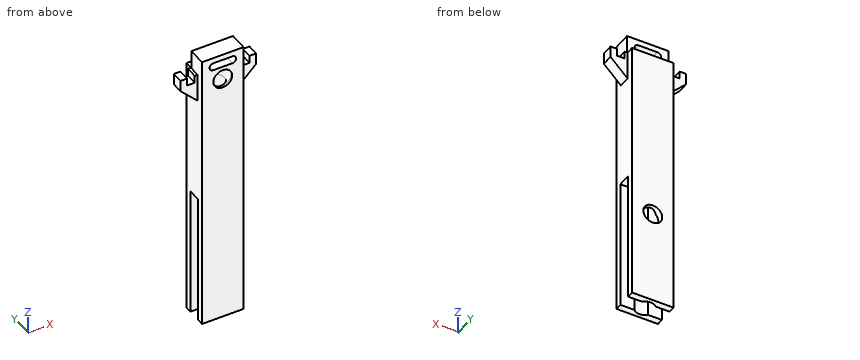
from build123d import *

# Parameters (mm, degrees)
SKETCH1_W           = 11
SKETCH1_H           = 76
BOSS_EXTRUDE1_DEPTH = 7
SKETCH4_R           = 2.5
SKETCH5_W           = 3
SKETCH5_H           = 3
BOSS_EXTRUDE2_DEPTH = 4.5
SKETCH6_W           = 2
SKETCH6_H           = 3
CUT_EXTRUDE2_DEPTH  = 2
BOSS_EXTRUDE3_DEPTH = 3
SKETCH10_W          = 11
SKETCH10_H          = 3.5
CUT_EXTRUDE5_DEPTH  = 35
CUT_EXTRUDE6_REACH  = 41.912
SKETCH11_R          = 2.5
SKETCH12_W          = 11
SKETCH12_H          = 2.25
CUT_EXTRUDE9_DEPTH  = 5
CUT_EXTRUDE10_REACH = 41.58


with BuildPart() as part:
    # Sketch1 → Boss-Extrude1 (new body)
    with BuildSketch(Plane(origin=(0, 0, 0), x_dir=(1, 0, 0), z_dir=(0, 1, 0))):
        Rectangle(SKETCH1_W, SKETCH1_H)
    extrude(amount=BOSS_EXTRUDE1_DEPTH)

    # Cut-Sweep2: sweep along a path in Sketch3
    with BuildLine(Plane.ZY) as cut_sweep2_path:
        Line((-38, 3.5), (28, 3.5))
        ThreePointArc((28, 3.5), (30.121320344, 2.621320344), (31, 0.5))
        Line((31, 0.5), (31, 0))
    # Sketch4 → Cut-Sweep2 (sweep, cut)
    with BuildSketch(Plane(origin=(0, 0, -38), x_dir=(-1, 0, 0), z_dir=(0, 0, -1))):
        with Locations((0, 3.5)):
            Circle(SKETCH4_R)
    sweep(path=cut_sweep2_path.line, mode=Mode.SUBTRACT)

    # Sketch5 → Boss-Extrude2 (add)
    with BuildSketch(Plane.ZY.offset(5.5)):
        with Locations((31.5, 3.5)):
            Rectangle(SKETCH5_W, SKETCH5_H)
    boss_extrude2 = extrude(amount=BOSS_EXTRUDE2_DEPTH)

    # Mirror1: Boss-Extrude2 across plane
    add(boss_extrude2.mirror(Plane.ZY))

    # Sketch6 → Cut-Extrude2 (cut)
    with BuildSketch(Plane.XY.offset(33)):
        with Locations((-7.25, 3.5)):
            Rectangle(SKETCH6_W, SKETCH6_H)
    cut_extrude2 = extrude(amount=-CUT_EXTRUDE2_DEPTH, mode=Mode.SUBTRACT)

    # Mirror2: Cut-Extrude2 across plane
    add(cut_extrude2.mirror(Plane.ZY), mode=Mode.SUBTRACT)

    # Sketch7 → Boss-Extrude3 (add)
    with BuildSketch(Plane(origin=(0, 5, 0), x_dir=(1, 0, 0), z_dir=(0, 1, 0))):
        Polygon((-10, -30), (-5.5, -25.5), (-5.5, -30), align=None)
    boss_extrude3 = extrude(amount=-BOSS_EXTRUDE3_DEPTH)

    # Mirror3: Boss-Extrude3 across plane
    add(boss_extrude3.mirror(Plane.ZY))

    # Sketch10 → Cut-Extrude5 (cut)
    with BuildSketch(Plane(origin=(0, 0, -38), x_dir=(-1, 0, 0), z_dir=(0, 0, -1))):
        with Locations((0, 3.5)):
            Rectangle(SKETCH10_W, SKETCH10_H)
    extrude(amount=-CUT_EXTRUDE5_DEPTH, mode=Mode.SUBTRACT)

    # Sketch11 → Cut-Extrude6 (cut, up to next)
    with BuildSketch(Plane(origin=(0, 7, 0), x_dir=(1, 0, 0), z_dir=(0, 1, 0)), mode=Mode.PRIVATE) as cut_extrude6_sk1:
        with Locations(Location((0, 13, 0), (0, 0, 270))):
            Circle(SKETCH11_R)
    cut_extrude6_tool1 = extrude(cut_extrude6_sk1.sketch, amount=-CUT_EXTRUDE6_REACH, mode=Mode.PRIVATE) & part.part
    add(cut_extrude6_tool1.solids().sort_by_distance((0, 7, -13))[0], mode=Mode.SUBTRACT)

    # Sketch12 → Cut-Extrude9 (cut)
    with BuildSketch(Plane.XY.offset(38)):
        with Locations((0, 5.875)):
            Rectangle(SKETCH12_W, SKETCH12_H)
    extrude(amount=-CUT_EXTRUDE9_DEPTH, mode=Mode.SUBTRACT)

    # Sketch14 → Cut-Extrude10 (cut, up to next)
    with BuildSketch(Plane(origin=(0, 4.75, 0), x_dir=(1, 0, 0), z_dir=(0, 1, 0)), mode=Mode.PRIVATE) as cut_extrude10_sk1:
        with BuildLine():
            Line((-2.5, -34.5), (2.5, -34.5))
            ThreePointArc((2.5, -34.5), (3.5, -35.5), (2.5, -36.5))
            Line((2.5, -36.5), (-2.5, -36.5))
            ThreePointArc((-2.5, -36.5), (-3.5, -35.5), (-2.5, -34.5))
        make_face()
    cut_extrude10_tool1 = extrude(cut_extrude10_sk1.sketch, amount=-CUT_EXTRUDE10_REACH, mode=Mode.PRIVATE) & part.part
    add(cut_extrude10_tool1.solids().sort_by_distance((0, 4.75, 35.5))[0], mode=Mode.SUBTRACT)


solid = part.part
The model under review builds one solid part; all positions refer to its coordinate system, in mm. Round coordinates to 2 decimals unless told otherwise and drop trailing zeros. Loops run counter-clockwise (first coordinate to the right, second up) from the corner with the lowest first, then second, coordinate; pieces in that order, holes last. Notation, with made-up numbers: (85, -38.75) - (107, -38.75) arc R33 ccw to (107, -7.75) - close; hole circle Ø11 at (36, 13). An arc over 180 degrees is marked (long way). Use CSV: the item, a comma, the result in double quotes.
(1) Take a section at A-A, the plane z = 35.5. Give the boundary of the cut face in (x, y), plus the area to 3 significant figures.
Working result:
outline,"(-5.5, 0) - (-3.5, 0) - (-3.5, 4.75) - (-5.5, 4.75) - close; (3.5, 0) - (5.5, 0) - (5.5, 4.75) - (3.5, 4.75) - close"
area,"19.0 mm^2"
(2) Take a section at C-C, the plane z = 4.5. Give the boundary of the cut face in (x, y).
Working result:
outline,"(-5.5, 0) - (5.5, 0) - (5.5, 7) - (-5.5, 7) - close; hole circle Ø5 at (0, 3.5)"
(3) Take a section at D-D, the plane x = -4.25. Give the boundary of the cut face in (y, z), plus the area to 3 significant figures.
Working result:
outline,"(0, -38) - (1.75, -38) - (1.75, -3) - (5.25, -3) - (5.25, -38) - (7, -38) - (7, 33) - (4.75, 33) - (4.75, 38) - (0, 38) - close"
area,"398 mm^2"
(4) For line 1 (Z direction, x = 0, y = 0.35); line 2 (Y direction, x = 0.25, z = 15.5); line 3 (Y direction, x = 5, z = -26), list the stretches that pass through material, from the lowest coordinate up.
Working result:
line 1,"z = -38 to 28.5, 33.5 to 34.5, 36.5 to 38"
line 2,"y = 0 to 1.01, 5.99 to 7"
line 3,"y = 0 to 1.75, 5.25 to 7"
(5) Clearance check with flat-ended pins moving along their axes: P1, Ø2, axis at x = 8.5, z = 29, coming from the -Y side; P2, Ø2, axis at x = 7, y = 3.5, coming from the +Z side; P3, Ø3.5, axis at x = 7.5, z = 30.5, coming from the +Y side. State where each tip first meets the part, or that it passes through.
Working result:
P1,"stops at y = 2"
P2,"stops at z = 33"
P3,"stops at y = 5"
(6) Take a section at B-B, the plane z = -13. Give the boundary of the cut face in (x, y), plus the area to 3 significant figures.
Working result:
outline,"(-5.5, 0) - (5.5, 0) - (5.5, 1.75) - (1.79, 1.75) arc R2.5 cw to (-1.79, 1.75) - (-5.5, 1.75) - close; (-5.5, 5.25) - (-2.5, 5.25) - (-2.5, 7) - (-5.5, 7) - close; (2.5, 5.25) - (5.5, 5.25) - (5.5, 7) - (2.5, 7) - close"
area,"27.9 mm^2"
